The listing builds one solid part. Answer for the finished solid, in the listing's coordinates (mm). Give positions to 0.01 mm unless a question says otherwise; leave off trailing zeros. Order: outer loops, then holes, each group sorted by start corner. A loop starts at its lowest first (then second) coordinate and runs counter-clockwise, first axis right, second up. Notation, with made-up numbers: M 43,17.25 L 88,17.25 A17 cw 88,26.25 Z; hole C -26,2 d7. An arc over 180 degrees is marked long. Answer as a JSON object with one key per item and string values. Group by question number.
```python
from build123d import *

# Parameters (mm, degrees)
BOSS_EXTRU_1_DEPTH                      = 7
ESQUISSE2_R                             = 4
ESQUISSE2_R_2                           = 1.2
BOSS_EXTRU_2_DEPTH                      = 7
CONG_1_R                                = 10
CONG_2_R                                = 3
BOSS_EXTRU_3_DEPTH                      = 41
ESQUISSE5_W                             = 29
ESQUISSE5_H                             = 22
ENL_V_MAT_EXTRU_1_DEPTH                 = 199.198296894
ESQUISSE7_W                             = 34
ESQUISSE7_H                             = 27
ENL_V_MAT_EXTRU_2_DEPTH                 = 7.4
ENL_V_START                             = -32
ESQUISSE8_W                             = 163.5
ESQUISSE8_H                             = 53
ENL_V_MAT_EXTRU_3_DEPTH                 = 170.279035308
ENL_V_MAT_EXTRU_4_DEPTH                 = 120.922123014
CONG_3_R                                = 3
DIAM_TRE_DU_PER_AGE_2_4_2_4_1_D         = 2.4
DIAM_TRE_DU_PER_AGE_2_4_2_4_1_ON_FACE_D = 2.4


with BuildPart() as part:
    # Esquisse1 → Boss.-Extru.1 (new body)
    with BuildSketch(Plane(origin=(0, 0, 0), x_dir=(1, 0, 0), z_dir=(0, 1, 0))):
        with BuildLine():
            Line((163.5, -54.314885969), (163.5, 54.839745962))
            Line((163.5, 54.839745962), (141, 93.810889132))
            Line((141, 93.810889132), (136.669872981, 91.310889132))
            Line((136.669872981, 91.310889132), (158.5, 53.5))
            Line((158.5, 53.5), (158.5, -53.5))
            ThreePointArc((158.5, -53.5), (146.077391865, -81.52236249), (128.750264504, -106.807627959))
            Line((128.750264504, -106.807627959), (132.598479772, -110))
            ThreePointArc((132.598479772, -110), (150.644566487, -83.59767596), (163.5, -54.314885969))
        make_face()
    extrude(amount=BOSS_EXTRU_1_DEPTH)

    # Esquisse2 → Boss.-Extru.2 (add)
    # profile 1 of 2: a face of its own
    with BuildSketch(Plane(origin=(0, 7, 0), x_dir=(1, 0, 0), z_dir=(0, 1, 0))):
        with Locations((155, 53)):
            Circle(ESQUISSE2_R)
        with Locations(Location((155, 53, 0), (0, 0, 270))):
            Circle(ESQUISSE2_R_2, mode=Mode.SUBTRACT)
    # profile 2 of 2: a face of its own
    with BuildSketch(Plane(origin=(0, 7, 0), x_dir=(1, 0, 0), z_dir=(0, 1, 0))):
        with Locations((140, -87)):
            Circle(ESQUISSE2_R)
        with Locations(Location((140, -87, 0), (0, 0, 270))):
            Circle(ESQUISSE2_R_2, mode=Mode.SUBTRACT)
    extrude(amount=-BOSS_EXTRU_2_DEPTH)

    # Congé1
    cong_1_edges = [part.edges().sort_by_distance(p)[0] for p in [
        (158.5, 3.5, 53.5),
        (163.5, 3.5, -54.839745962),
        (163.5, 3.5, 54.314885969),
    ]]
    fillet(cong_1_edges, radius=CONG_1_R)

    # Congé2
    cong_2_edges = [part.edges().sort_by_distance(p)[0] for p in [
        (128.750264504, 3.5, 106.807627959),
        (156.697559724, 3.5, -56.621918136),
        (158.5, 3.5, -51.063508327),
        (140.380940937, 3.5, 90.981819183),
        (143.738827918, 3.5, 85.578322891),
    ]]
    fillet(cong_2_edges, radius=CONG_2_R)

    # Esquisse4 → Boss.-Extru.3 (add)
    with BuildSketch(Plane(origin=(0, 7, 0), x_dir=(1, 0, 0), z_dir=(0, 1, 0))):
        with BuildLine():
            Line((162.160254038, 57.160254038), (141, 93.810889132))
            Line((141, 93.810889132), (133.205771366, 89.310889132))
            Line((133.205771366, 89.310889132), (153.015172443, 55))
            Line((153.015172443, 55), (155, 55))
            ThreePointArc((155, 55), (156, 54.732050808), (156.732050808, 54))
            Line((156.732050808, 54), (158.5, 50.937822174))
            Line((158.5, 50.937822174), (158.5, 33))
            Line((158.5, 33), (163.5, 33))
            Line((163.5, 33), (163.5, 52.160254038))
            ThreePointArc((163.5, 52.160254038), (163.159258263, 54.748444489), (162.160254038, 57.160254038))
        make_face()
    extrude(amount=-BOSS_EXTRU_3_DEPTH)

    # Esquisse5 → Enlèv. mat.-Extru.1 (cut, through all)
    with BuildSketch(Plane(origin=(146.37130657, 0, -84.50751325), x_dir=(-0.4999999999999999, 0, -0.8660254037844387), z_dir=(0.8660254037844387, 0, -0.4999999999999999))):
        with Locations((-10.417640898, -13.5)):
            Rectangle(ESQUISSE5_W, ESQUISSE5_H)
    extrude(amount=-ENL_V_MAT_EXTRU_1_DEPTH, mode=Mode.SUBTRACT)

    # Esquisse7 → Enlèv. mat.-Extru.2 (cut)
    with BuildSketch(Plane(origin=(146.37130657, 0, -84.50751325), x_dir=(-0.4999999999999999, 0, -0.8660254037844387), z_dir=(0.8660254037844387, 0, -0.4999999999999999))):
        with Locations((-10.417640898, -13.5)):
            Rectangle(ESQUISSE7_W, ESQUISSE7_H)
    extrude(amount=-ENL_V_MAT_EXTRU_2_DEPTH, mode=Mode.SUBTRACT)

    # Esquisse8 → Enlèv. mat.-Extru.3 (cut, through all)
    with BuildSketch(Plane(origin=(0, 7, 0), x_dir=(1, 0, 0), z_dir=(0, 1, 0)).offset(ENL_V_START)):
        with Locations((81.75, 26.5)):
            Rectangle(ESQUISSE8_W, ESQUISSE8_H)
    extrude(amount=-ENL_V_MAT_EXTRU_3_DEPTH, mode=Mode.SUBTRACT)

    # Esquisse9 → Enlèv. mat.-Extru.4 (cut, through all)
    with BuildSketch(Plane(origin=(163.5, 0, 0), x_dir=(0, 0, -1), z_dir=(1, 0, 0))):
        with BuildLine():
            Line((60.763139721, -11.5), (48.390964663, -11.5))
            ThreePointArc((48.390964663, -11.5), (37.25, -13.5), (48.390964663, -15.5))
            Line((48.390964663, -15.5), (60.763139721, -15.5))
            Line((60.763139721, -15.5), (60.763139721, -11.5))
        make_face()
    extrude(amount=-ENL_V_MAT_EXTRU_4_DEPTH, mode=Mode.SUBTRACT)

    # Congé3
    cong_3_edges = [part.edges().sort_by_distance(p)[0] for p in [
        (133.205771366, -13.5, -89.310889132),
    ]]
    fillet(cong_3_edges, radius=CONG_3_R)

    # Diamètre du perçage Ø2.4 (2.4)1 (through all)
    with Locations(Plane(origin=(135.734675085, 3, 106.105866084), x_dir=(-0.615871636874, 0, 0.787846512269), z_dir=(0.787846512269, 0, 0.615871636874))):
        with Locations((0, 0)):
            Hole(DIAM_TRE_DU_PER_AGE_2_4_2_4_1_D / 2)

    # Diamètre du perçage Ø2.4 (2.4)1 on face (through all)
    with Locations(Plane(origin=(163.5, 3, -45), x_dir=(0, 0, 1), z_dir=(1, 0, 0))):
        with Locations((0, 0), (90, 0)):
            Hole(DIAM_TRE_DU_PER_AGE_2_4_2_4_1_ON_FACE_D / 2)


solid = part.part
```
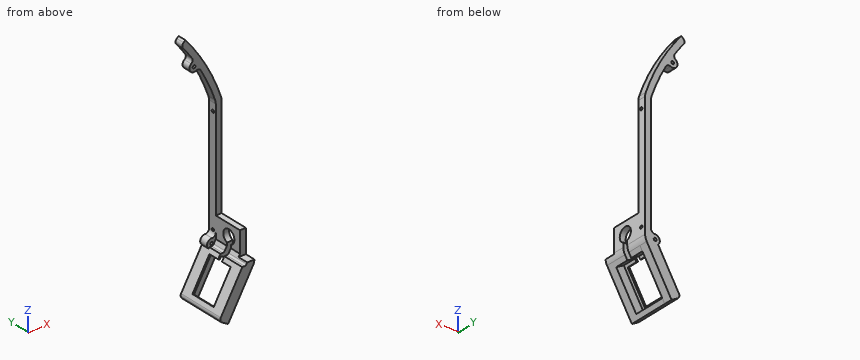
Item 1: Section A-A (z = -65) is taken. Determine the outline of the cut face in (x, y).
Item 2: Section B-B (z = 36.5) is taken. Determine the outline of the cut face in (x, y), and give its area (3 significant figures).
Item 3: Flat-ended cylindrical pins translate along their axes: P1, Ø0.6, axis at x = 154, y = -26, coming from the +Z side; P2, Ø1.9, axis at x = 155, z = -53, coming from the +Y side; P3, Ø5.5, axis at x = 160, y = -16.5, coming from the +Z side; P4, Ø5, axis at x = 159, z = -43, coming from the -Y side. Find the tip coordinate at first contact, or state that the pin passes through.
Item 4: Consider probe 1 along X at (y, z) = (2.75, -53); probe 2 along Z at (x, y) = (140, 2); probe 3 along Y at (x, z) = (161, -45). Determine where each line is inside the solid, lowest interval first. Write a range as from..to.
Values found:
{
 "1": {"outline": "M 147.24,-34 L 157.63,-34 L 157.63,-27 L 149.09,-27 L 149.09,-24.5 L 147.24,-24.5 Z; M 147.24,-2.5 L 149.09,-2.5 L 149.09,0 L 157.63,0 L 157.63,7 L 147.24,7 Z"},
 "2": {"outline": "M 158.5,0 L 163.5,0 L 163.5,7 L 158.5,7 Z", "area": "35.0 mm^2"},
 "3": {"P1": "stops at z = -55", "P2": "passes through", "P3": "stops at z = -33", "P4": "stops at y = -25"},
 "4": {"probe 1": "x = 151..153.8, 156.2..163.46", "probe 2": "z = -93.23..-77.54, 83..85.8, 88.2..100.41", "probe 3": "y = -25..-18.89, -8.11..1.8, 4.2..7"}
}
